Model file for the job. Use its own axes, mm. Face numbers are marked on the shaded views. A direction names the side the tool comes from. Round coordinates to 2 decimals unless told otherwise and drop trailing zeros. Loops run counter-clockwise (first coordinate to the right, second up) from the corner with the lowest first, then second, coordinate; pieces in that order, holes last. Notation, with made-up numbers: M 16,0 L 59,0 A22 cw 59,27 Z; hole C -39.75,46.25 d6. An arc over 180 degrees is marked long. Use a Markdown table: item, result. Add a question column.
Q1. Cut at B-B (z = 52). Give the cut face in (x, y), plus the area to 3 significant figures.
Q2. Tool access for the marked faces 5 and 6: list every direction of +Z, -Z, +X, -X, +Y, -Y with a clear straight run to the whole face (end or side of a thin tool).
Q3. Pin check, flat tips, straight feed: pin 1 (11 mm diameter, centred on x = -8.47, z = 12.5, fed in from -Y); pin 2 (3 mm diameter, centred on y = 3.5, z = 38.5, fed in from +X); pin 3 (5.5 mm diameter, centred on x = -18, z = 29, fed in from +Y); pin 4 (5 mm diameter, centred on x = -43, z = 52, fed in from +Y). Stop position of each tip, or through.
Q4. Cut at A-A (x = -82.5). Give the cut face in (y, z).
Q5. Probe line 1 (Z direction, x = -18, y = 3.5); line 2 (Z direction, x = -91.5, y = 3); line 3 (X direction, y = 9.25, z = 18.5). List the from-to ranges inside material, lowest first. Write a range as from..to.
Q6. Mould opens along Z. For the marked faces 1, 2, 3 and 4 say: +Z half, -Z half, draft (parallel to the pull), parting line (faces both ways), or undercut.
Q7. Cut at C-C (x = -43). Give the cut face in (y, z).
Autodesk Inventor part; units mm, degrees
ref_plane "YZ Plane" through (0, 0, 0) normal (1, 0, 0) x (0, 1, 0)
ref_plane "XZ Plane" through (0, 0, 0) normal (0, 1, 0) x (-1, 0, 0)
ref_plane "XY Plane" through (0, 0, 0) normal (0, 0, 1) x (1, 0, 0)
sketch "Esquisse1" plane through (0, 0, 0) normal (0, 1, 0) x (-1, 0, 0)
  line L0 (0, 0) -> (123, 0)
  line L1 (123, 0) -> (123, 60)
  line L2 (123, 60) -> (0, 60)
  line L3 (0, 60) -> (0, 0)
  dimension "d1" = 123
  dimension "d2" = 60
extrude "Extrusion1" add sketch "Esquisse1" along normal blind 10
sketch "Esquisse2" plane through (0, 10, 0) normal (0, 1, 0) x (1, 0, 0)
  circle A0 centre (-18, -18) radius 9
  line L0 (0, 0) -> (-123, 0)
  line L1 (-123, 0) -> (-123, -60)
  line L2 (-123, -60) -> (0, -60)
  line L3 (0, -60) -> (0, 0)
  line L4 (-29, -9) -> (-7, -9) construction
  line L5 (-7, -9) -> (-7, -56) construction
  line L6 (-7, -56) -> (-29, -56) construction
  line L7 (-29, -56) -> (-29, -9) construction
  dimension "d5" = 18
  dimension "d7" = 18
  dimension "d9" = 18
  dimension "d27" = 22
  dimension "d28" = 11
  dimension "d29" = 9
  dimension "d30" = 47
  dimension "d31" = 7
  dimension "d44" = 9
extrude "Extrusion2" cut sketch "Esquisse2" against normal up to surface (10 mm away) contours A0
sketch "Esquisse4" plane through (0, 10, 0) normal (0, 1, 0) x (1, 0, 0)
  circle A0 centre (-18, -18) radius 9
  line L0 (0, 0) -> (-123, 0)
  line L1 (-123, 0) -> (-123, -60)
  line L2 (-123, -60) -> (0, -60)
  line L3 (0, -60) -> (0, 0)
  point P0 (-18, -29)
  dimension "d16" = 11
hole "Perçage1" at (-18, 10, 29) direction (0, -1, 0) diameter 3.4 end through all counterbore diameter 7 counterbore depth 4
pattern_circular "Réseau circulaire1" count 3 over 360 about axis through (-18, 10, 18) along (0, -1, 0) of "Perçage1"
sketch "Esquisse5" plane through (0, 10, 0) normal (0, 1, 0) x (1, 0, 0)
  arc A0 (-9.2451, -15.9139) -> (-11.816, -11.4611) centre (-8.4737, -12.5) ccw
  arc A1 (-15.4291, -26.625) -> (-9.2451, -15.9139) centre (-18, -18) ccw
  arc A2 (-20.5709, -26.625) -> (-15.4291, -26.625) centre (-18, -29) ccw
  arc A3 (-26.7549, -15.9139) -> (-20.5709, -26.625) centre (-18, -18) ccw
  arc A4 (-24.184, -11.4611) -> (-26.7549, -15.9139) centre (-27.5263, -12.5) ccw
  arc A5 (-11.816, -11.4611) -> (-24.184, -11.4611) centre (-18, -18) ccw
  line L0 (0, 0) -> (-123, 0)
  line L1 (-123, 0) -> (-123, -60)
  line L2 (-123, -60) -> (0, -60)
  line L3 (0, -60) -> (0, 0)
  line L4 (-29, -18.7209) -> (-29, -39.8718) construction
  point P0 (-43, -8)
  point P1 (-43, -52)
  point P2 (-107, -8)
  point P3 (-107, -52)
  dimension "d32" = 11
  dimension "d33" = 14
  dimension "d34" = 8
  dimension "d35" = 8
  dimension "d36" = 16
hole "Perçage2" at (-43, 10, 8) at (-43, 10, 52) at (-107, 10, 8) at (-107, 10, 52) direction (0, -1, 0) diameter 5.5 end through all
sketch "Esquisse6" plane through (0, 10, 0) normal (0, 1, 0) x (1, 0, 0)
  circle A0 centre (-107, -8) radius 2.75
  circle A1 centre (-43, -8) radius 2.75
  circle A2 centre (-43, -52) radius 2.75
  circle A3 centre (-107, -52) radius 2.75
  arc A4 (-9.2451, -15.9139) -> (-11.816, -11.4611) centre (-8.4737, -12.5) ccw
  arc A5 (-15.4291, -26.625) -> (-9.2451, -15.9139) centre (-18, -18) ccw
  arc A6 (-20.5709, -26.625) -> (-15.4291, -26.625) centre (-18, -29) ccw
  arc A7 (-26.7549, -15.9139) -> (-20.5709, -26.625) centre (-18, -18) ccw
  arc A8 (-24.184, -11.4611) -> (-26.7549, -15.9139) centre (-27.5263, -12.5) ccw
  arc A9 (-11.816, -11.4611) -> (-24.184, -11.4611) centre (-18, -18) ccw
  line L0 (0, 0) -> (-123, 0)
  line L1 (-123, 0) -> (-123, -60)
  line L2 (-123, -60) -> (0, -60)
  line L3 (0, -60) -> (0, 0)
  line L4 (-99, -10) -> (-78, -10)
  line L5 (-78, -10) -> (-78, -27)
  line L6 (-78, -27) -> (-99, -27)
  line L7 (-99, -27) -> (-99, -10)
  line L8 (-72, -10) -> (-51, -10)
  line L9 (-51, -10) -> (-51, -27)
  line L10 (-51, -27) -> (-72, -27)
  line L11 (-72, -27) -> (-72, -10)
  line L12 (-72, -33) -> (-51, -33)
  line L13 (-51, -33) -> (-51, -50)
  line L14 (-51, -50) -> (-72, -50)
  line L15 (-72, -50) -> (-72, -33)
  line L16 (-99, -33) -> (-78, -33)
  line L17 (-78, -33) -> (-78, -50)
  line L18 (-78, -50) -> (-99, -50)
  line L19 (-99, -50) -> (-99, -33)
  dimension "d47" = 10
  dimension "d48" = 10
  dimension "d49" = 8
  dimension "d50" = 6
  dimension "d51" = 6
  dimension "d52" = 8
extrude "Extrusion4" cut sketch "Esquisse6" against normal up to surface (10 mm away) contours L4 L5 L6 L7 | L8 L9 L10 L11 | L12 L13 L14 L15 | L16 L17 L18 L19
chamfer "Chanfrein1" distance 2 angle 45 16 edges at (-78, 5, 27) (-78, 5, 50) (-51, 5, 50) (-51, 5, 27) (-72, 5, 33) (-72, 5, 10) (-99, 5, 10) (-99, 5, 33) (-78, 5, 33) (-78, 5, 10) (-51, 5, 10) (-51, 5, 33) (-99, 5, 50) (-72, 5, 50) (-99, 5, 27) (-72, 5, 27)
sketch "Esquisse7" plane through (0, 10, 0) normal (0, 1, 0) x (1, 0, 0)
  line L0 (0, 0) -> (-123, 0)
  line L1 (-101, 0) -> (-49, 0)
  line L2 (-49, 0) -> (-49, -60)
  line L3 (-49, -60) -> (-101, -60)
  line L4 (-101, -60) -> (-101, 0)
  line L5 (-51, -35) -> (-51, -48)
  line L6 (-53, -50) -> (-51, -48)
  line L7 (-53, -50) -> (-70, -50)
  line L8 (-72, -48) -> (-70, -50)
  line L9 (-72, -48) -> (-72, -35)
  line L10 (-70, -33) -> (-72, -35)
  line L11 (-70, -33) -> (-53, -33)
  line L12 (-51, -35) -> (-53, -33)
  line L13 (-80, -50) -> (-97, -50)
  line L14 (-99, -48) -> (-97, -50)
  line L15 (-99, -48) -> (-99, -35)
  line L16 (-97, -33) -> (-99, -35)
  line L17 (-97, -33) -> (-80, -33)
  line L18 (-78, -35) -> (-80, -33)
  line L19 (-78, -35) -> (-78, -48)
  line L20 (-80, -50) -> (-78, -48)
  line L21 (-51, -12) -> (-51, -25)
  line L22 (-53, -27) -> (-51, -25)
  line L23 (-53, -27) -> (-70, -27)
  line L24 (-72, -25) -> (-70, -27)
  line L25 (-72, -25) -> (-72, -12)
  line L26 (-70, -10) -> (-72, -12)
  line L27 (-70, -10) -> (-53, -10)
  line L28 (-51, -12) -> (-53, -10)
  line L29 (-80, -27) -> (-97, -27)
  line L30 (-99, -25) -> (-97, -27)
  line L31 (-99, -25) -> (-99, -12)
  line L32 (-97, -10) -> (-99, -12)
  line L33 (-97, -10) -> (-80, -10)
  line L34 (-78, -12) -> (-80, -10)
  line L35 (-78, -12) -> (-78, -25)
  line L36 (-80, -27) -> (-78, -25)
  circle A0 centre (-107, -8) radius 2.75
  circle A1 centre (-43, -8) radius 2.75
  circle A2 centre (-43, -52) radius 2.75
  circle A3 centre (-107, -52) radius 2.75
  arc A4 (-9.2451, -15.9139) -> (-11.816, -11.4611) centre (-8.4737, -12.5) ccw
  arc A5 (-15.4291, -26.625) -> (-9.2451, -15.9139) centre (-18, -18) ccw
  arc A6 (-20.5709, -26.625) -> (-15.4291, -26.625) centre (-18, -29) ccw
  arc A7 (-26.7549, -15.9139) -> (-20.5709, -26.625) centre (-18, -18) ccw
  arc A8 (-24.184, -11.4611) -> (-26.7549, -15.9139) centre (-27.5263, -12.5) ccw
  arc A9 (-11.816, -11.4611) -> (-24.184, -11.4611) centre (-18, -18) ccw
  line L37 (0, -60) -> (0, 0)
  line L38 (0, 0) -> (-123, 0)
  line L39 (-123, 0) -> (-123, -60)
  line L40 (-123, -60) -> (0, -60)
  line L41 (-123, -60) -> (-25, -60)
  point P0 (-5, 0)
  dimension "d67" = 6
  dimension "d68" = 6
extrude "Extrusion5" cut sketch "Esquisse7" against normal blind 4 contours L2 L3 L4 L0
chamfer "Chanfrein5" distance 2 angle 45 2 edges at (-101, 6, 30) (-49, 6, 30)
sketch "Esquisse8" plane through (0, 10, 0) normal (0, 1, 0) x (1, 0, 0)
  line L0 (-123, -60) -> (0, -60)
  line L1 (0, -60) -> (-25, -60)
  line L2 (-25, -60) -> (-25, -38)
  line L3 (-25, -38) -> (0, -38)
  line L4 (0, -38) -> (0, -60)
  point P0 (0, 0)
  dimension "d74" = 25
  dimension "d75" = 22
extrude "Extrusion6" cut sketch "Esquisse8" against normal up to surface (10 mm away)
chamfer "Chanfrein6" distance 4 angle 45 2 edges at (-25, 5, 38) (-25, 5, 60)
chamfer "Chanfrein7" distance 8 angle 45 2 edges at (0, 5, 38) (0, 5, 0)
equation "\"d28\" = 0.5 * d27"
equation "\"d51\" = d50"
properties part number "attache_moteur"
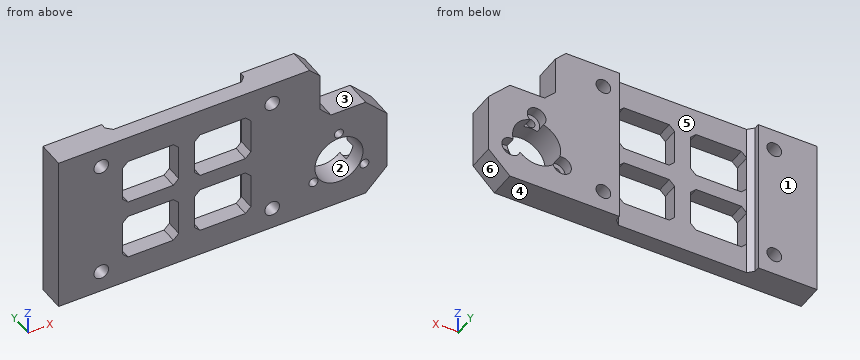
Checked values:
| question | item | result |
|---|---|---|
| 1 | outline | M -123,0 L -109.75,0 L -109.75,10 L -123,10 Z; M -104.25,0 L -45.75,0 L -45.75,10 L -49,10 L -49,8 L -51,6 L -99,6 L -101,8 L -101,10 L -104.25,10 Z; M -40.25,0 L -25,0 L -25,10 L -40.25,10 Z |
| 1 | area | 666 mm^2 |
| 2 | face 5 | +Z, -Z, +Y |
| 2 | face 6 | -Z, +X, +Y, -Y |
| 3 | pin 1 | stops at y = 0 |
| 3 | pin 2 | stops at x = -7 |
| 3 | pin 3 | stops at y = 6 |
| 3 | pin 4 | passes through |
| 4 | outline | M 0,0 L 6,0 L 6,10 L 0,10 Z; M 0,27 L 6,27 L 6,33 L 0,33 Z; M 0,50 L 6,50 L 6,60 L 0,60 Z |
| 5 | line 1 | z = 0..9, 27..27.3, 30.7..38 |
| 5 | line 2 | z = 0..10, 27..33, 50..60 |
| 5 | line 3 | x = -123..-101, -49..-26.99, -9.01..0 |
| 6 | face 1 | draft |
| 6 | face 2 | undercut |
| 6 | face 3 | +Z half |
| 6 | face 4 | -Z half |
| 7 | outline | M 0,0 L 10,0 L 10,5.25 L 0,5.25 Z; M 0,10.75 L 10,10.75 L 10,49.25 L 0,49.25 Z; M 0,54.75 L 10,54.75 L 10,60 L 0,60 Z |
